from build123d import *

# Parameters (mm, degrees)
SKETCH1_R           = 6.35
SKETCH1_R_2         = 3.175
SKETCH1_W           = 40.64
SKETCH1_H           = 20.32
BOSS_EXTRUDE1_DEPTH = 5.0038
SKETCH2_R           = 10.425848265
SKETCH2_R_2         = 2.159
SKETCH2_R_3         = 8.142875018
BOSS_EXTRUDE2_DEPTH = 5.0038
SKETCH3_R           = 0.50000027
CUT_EXTRUDE1_DEPTH  = 19.304


with BuildPart() as part:
    # Sketch1 → Boss-Extrude1 (new body)
    with BuildSketch(Plane.XY):
        with BuildLine():
            ThreePointArc((108.923032041, -12.7), (114.491880219, -7.405308906), (116.543032041, 0))
            Line((116.543032041, 0), (116.543032041, 40.64))
            Line((116.543032041, 40.64), (55.583032041, 40.64))
            Line((55.583032041, 40.64), (55.583032041, 12.7))
            Line((55.583032041, 12.7), (-152.4, 12.7))
            ThreePointArc((-152.4, 12.7), (-165.1, 0), (-152.4, -12.7))
            Line((-152.4, -12.7), (108.923032041, -12.7))
        make_face()
        with Locations((-152.4, 0)):
            Circle(SKETCH1_R, mode=Mode.SUBTRACT)
        Circle(SKETCH1_R_2, mode=Mode.SUBTRACT)
        with Locations((101.6, 0)):
            Circle(SKETCH1_R, mode=Mode.SUBTRACT)
        with Locations((88.603032041, 22.86)):
            Rectangle(SKETCH1_W, SKETCH1_H, mode=Mode.SUBTRACT)
    extrude(amount=BOSS_EXTRUDE1_DEPTH)

    # Sketch2 → Boss-Extrude2 (add)
    with BuildSketch(Plane.XY.offset(5.0038)):
        with Locations((-152.4, 0)):
            Circle(SKETCH2_R)
        with Locations((-152.4, 0)):
            Circle(SKETCH2_R_2, mode=Mode.SUBTRACT)
        with Locations((101.6, 0)):
            Circle(SKETCH2_R_3)
        with Locations((101.6, 0)):
            Circle(SKETCH2_R_2, mode=Mode.SUBTRACT)
    extrude(amount=-BOSS_EXTRUDE2_DEPTH)

    # Sketch3 → Cut-Extrude1 (cut)
    with BuildSketch(Plane(origin=(0, 0, 0), x_dir=(-1, 0, 0), z_dir=(0, 0, -1))):
        with Locations((16.5354, 0)):
            Circle(SKETCH3_R)
        with Locations((-16.5354, 0)):
            Circle(SKETCH3_R)
    extrude(amount=-CUT_EXTRUDE1_DEPTH, mode=Mode.SUBTRACT)


solid = part.part
Input: part model. Units: mm. Frame: model coordinates. A direction names the side the tool comes from. Coordinates: 2 decimals unless noted, no trailing zeros. Write each loop counter-clockwise with the first axis right and the second up, starting at its lowest first coordinate (ties: lowest second). Pieces come first, ordered by that corner, then holes. Notation, with made-up numbers: M 69,52.5 L 95,52.5 A22 ccw 95,76.5 Z; hole C 34.25,88 d6. An arc over 180 degrees is marked long. Answer as a JSON object with one key per item and string values. Group by question number.
(1) Ray query, line 1 along Y through (x, z) = (101.6, 1.6); line 2 along X through (y, z) = (29, 3.8); line 3 along Y through (x, z) = (86.5, 1.85). Return the intervals inside material, ascending. Write a range as [from, to].
(2) Section A-A on y = 20. Output: boundary loops of the cut face in (x, z), plus the area to 3 significant figures.
(3) Set-up query: faces 1 (the face through (-26, 2, 0)), 2 (the face through (68.283, 23, 2)), 3 (the face through (55.583, 27, 2)). Return all of +Z, -Z, +X, -X, +Y, -Y with unobstructed straight access to the full face (end or side cutting, diameter ignored); none if empty.
(4) Section D-D on x = -100.5. Output: boundary loops of the cut face in (y, z).
(5) Section C-C on z = 4.05. Output: boundary loops of the cut face in (x, y) (3 decimals), plus the area to 3 significant figures.
(6) Contact query for flat-ended pins moving along their axis: P1, Ø7.5, axis at x = 0, y = 0, coming from the +Z side; P2, Ø1.5, axis at y = 23, z = 3.5, coming from the -X side; P3, Ø1.5, axis at x = 19.5, z = 4, coming from the +Y side; P4, Ø3, axis at y = 12, z = 4, coming from the -X side. Output: stop coordinate, or through.
(7) Section B-B on x = 0. Output: boundary loops of the cut face in (y, z) (3 decimals), plus the area to 3 significant figures.
(8) Mould query, pull axis Y, two halves, no side actions, for faces 4 (the face through (-165.097, 0.279, 2.467)), 5 (the face through (-47, 12.7, 2)), 6 (the face through (-0.69, -3.1, 2.47)), 7 (the face through (116.543, 20, 2)). Classes: pulls with the +Y half, pulls with the -Y half, needs draft (parallel to the pull), parting line crosses it, or undercut.
Result set:
{
 "1": {"line 1": "y = [-12.7, -2.16], [2.16, 12.7], [33.02, 40.64]", "line 2": "x = [55.58, 68.28], [108.92, 116.54]", "line 3": "y = [-12.7, 12.7], [33.02, 40.64]"},
 "2": {"outline": "M 55.58,0 L 68.28,0 L 68.28,5 L 55.58,5 Z; M 108.92,0 L 116.54,0 L 116.54,5 L 108.92,5 Z", "area": "102 mm2"},
 "3": {"face 1": "-Z, +X, -X, +Y, -Y", "face 2": "+Z, -Z", "face 3": "+Z, -Z, -X, +Y"},
 "4": {"outline": "M -12.7,0 L 12.7,0 L 12.7,5 L -12.7,5 Z"},
 "5": {"outline": "M -152.4,-12.7 L 108.923,-12.7 A14.393 ccw 116.543,0 L 116.543,40.64 L 55.583,40.64 L 55.583,12.7 L -152.4,12.7 A12.7 ccw Z; hole C -152.4,0 d4.318; hole C -16.535,0 d1; hole C 0,0 d6.35; hole C 16.535,0 d1; hole M 68.283,12.7 L 108.923,12.7 L 108.923,33.02 L 68.283,33.02 Z; hole C 101.6,0 d4.318", "area": "7,870 mm2"},
 "6": {"P1": "stops at z = 5", "P2": "stops at x = 55.58", "P3": "stops at y = 12.7", "P4": "stops at x = -159.54"},
 "7": {"outline": "M -12.7,0 L -3.175,0 L -3.175,5.004 L -12.7,5.004 Z; M 3.175,0 L 12.7,0 L 12.7,5.004 L 3.175,5.004 Z", "area": "95.3 mm2"},
 "8": {"face 4": "parting line crosses it", "face 5": "pulls with the +Y half", "face 6": "undercut", "face 7": "needs draft"}
}
